Input: part model. Units: mm. Frame: model coordinates. A direction names the side the tool comes from. Coordinates: 2 decimals unless noted, no trailing zeros. Loops run counter-clockwise (first coordinate to the right, second up) from the corner with the lowest first, then second, coordinate; pieces in that order, holes last.
```python
from build123d import *
from build123d.topology import SkipClean

# Parameters (mm, degrees)
SKETCH1_R               = 31
SKETCH1_R_2             = 27.5
BOSS_EXTRUDE1_DEPTH     = 62
BOSS_EXTRUDE3_START     = 5
BOSS_EXTRUDE3_DEPTH     = 5
CUT_EXTRUDE1_DEPTH      = 76.934182026
CUT_EXTRUDE1_DEPTH_BACK = 76.934182026
SKETCH8_W               = 15
SKETCH8_H               = 52
SKETCH9_R               = 13.5
SKETCH9_R_2             = 11
BOSS_EXTRUDE4_DEPTH     = 26
SKETCH10_R              = 13.5
BOSS_EXTRUDE5_DEPTH     = 3
SKETCH12_R              = 1.5
CUT_EXTRUDE2_DEPTH      = 3


with BuildPart() as part:
    # Sketch1 → Boss-Extrude1 (new body)
    with BuildSketch(Plane(origin=(0, 0, 0), x_dir=(1, 0, 0), z_dir=(0, 1, 0))):
        with Locations(Location((0, 0, 0), (0, 0, 270))):
            Circle(SKETCH1_R)
        with Locations(Location((0, 0, 0), (0, 0, 270))):
            Circle(SKETCH1_R_2, mode=Mode.SUBTRACT)
    extrude(amount=BOSS_EXTRUDE1_DEPTH)

    # Sketch6 → Boss-Extrude3 (add)
    with SkipClean():  # the faces are left unmerged after this step: merging them gives an invalid solid
        with BuildSketch(Plane.XZ.offset(BOSS_EXTRUDE3_START)):
            with BuildLine():
                Line((31, 0), (27.5, 0))
                ThreePointArc((27.5, 0), (27.395354198, -2.396782926), (27.082213208, -4.775324886))
                Line((27.082213208, -4.775324886), (30.529040343, -5.383093508))
                ThreePointArc((30.529040343, -5.383093508), (30.882035641, -2.701828025), (31, 0))
            make_face()
            with BuildLine():
                ThreePointArc((27.082213208, 4.775324886), (27.395354198, 2.396782926), (27.5, 0))
                Line((27.5, 0), (31, 0))
                ThreePointArc((31, 0), (30.882035641, 2.701828025), (30.529040343, 5.383093508))
                Line((30.529040343, 5.383093508), (27.082213208, 4.775324886))
            make_face()
        extrude(amount=-BOSS_EXTRUDE3_DEPTH)

    # Sketch8 → Cut-Extrude1 (cut, two sides: drawn at the far end of the back side and taken through both)
    with BuildSketch(Plane.XY.offset(-CUT_EXTRUDE1_DEPTH_BACK)):
        with Locations((0, 31)):
            Rectangle(SKETCH8_W, SKETCH8_H)
    extrude(amount=CUT_EXTRUDE1_DEPTH + CUT_EXTRUDE1_DEPTH_BACK, mode=Mode.SUBTRACT)

    # Sketch9 → Boss-Extrude4 (add)
    with BuildSketch(Plane(origin=(-7.5, 0, 0), x_dir=(0, 0, -1), z_dir=(1, 0, 0))):
        with Locations(Location((41.079062485, 29.5, 0), (0, 0, 270))):
            Circle(SKETCH9_R)
        with Locations((41.079062485, 29.5)):
            Circle(SKETCH9_R_2, mode=Mode.SUBTRACT)
    boss_extrude4 = extrude(amount=-BOSS_EXTRUDE4_DEPTH)

    # Sketch10 → Boss-Extrude5 (add)
    with BuildSketch(Plane.ZY.offset(33.5)):
        with Locations(Location((-41.079062485, 29.5, 0), (0, 0, 270))):
            Circle(SKETCH10_R)
    boss_extrude5 = extrude(amount=BOSS_EXTRUDE5_DEPTH)

    # Sketch12 → Cut-Extrude2 (cut)
    with BuildSketch(Plane(origin=(-17.285590039, -28.448353543, -28.838033475), x_dir=(1, 0, 0), z_dir=(0, 0, 1))):
        with Locations((-14.214409961, 57.948353543)):
            Circle(SKETCH12_R)
    cut_extrude2 = extrude(amount=-CUT_EXTRUDE2_DEPTH, mode=Mode.SUBTRACT)

    # Mirror1: Boss-Extrude4, Boss-Extrude5, Cut-Extrude2 across plane
    add(boss_extrude4.mirror(Plane.XY))
    add(boss_extrude5.mirror(Plane.XY))
    add(cut_extrude2.mirror(Plane.XY), mode=Mode.SUBTRACT)


solid = part.part
```
Item 1: Mould query, pull axis X, two halves, no side actions, for faces 1 (the face through (-20.32, 25.29, 51.24)), 2 (the face through (7.5, 31, 28)), 3 (the face through (-36.5, 30, -41)), 4 (the face through (0, 57, 29)). Classes: +X half, -X half, draft (parallel to the pull), parting line (faces both ways), or undercut.
Result:
face 1: draft
face 2: undercut
face 3: -X half
face 4: undercut
Item 2: Contact query for flat-ended pins moving along their axis: P1, Ø11, axis at y = 34, z = -39, coming from the +X side; P2, Ø3, axis at y = 19, z = -29, coming from the -X side; P3, Ø8, axis at x = 13, y = 54, coming from the +Z side; P4, Ø18.5, axis at x = 0.5, z = 9.5, coming from the -Y side. Output: stop coordinate, or through.
Result:
P1: stops at x = -33.5
P2: stops at x = -14.31
P3: stops at z = 29.66
P4: passes through
Item 3: Reachability of faces 5 (the face through (0, 57, -29)), 6 (the face through (-20.32, 25.29, -51.24)), 7 (the face through (-33, 29.57, 29.5)) from +Z, -Z, +X, -X, +Y, -Y: full face, straight path, thin tool, end or side. Return the list, or none.
Result:
face 5: +Z, -Z
face 6: +X
face 7: none
Item 4: Line query: L1, parallel to Z at x = -9, y = 25.5; L2, parallel to Z at x = -33, y = 25.5; L3, parallel to X at y = 18, z = 0. Output: solid intervals per line, ascending.
Result:
L1: z = -53.97 to -51.33, -30.83 to -25.99, 25.99 to 30.83, 51.33 to 53.97
L2: z = -53.97 to -51.33, -30.83 to -28.19, 28.19 to 30.83, 51.33 to 53.97
L3: x = -31 to -27.5, 27.5 to 31
Item 5: Section query A-A (y = 13). Output: boundary loops of the cut face in (x, z), then the cut area to 3 significant figures.
Result:
outline: (-7.5, -30.08) - (-7.5, -26.46) arc R27.5 cw to (-7.5, 26.46) - (-7.5, 30.08) arc R31 ccw to start; (7.5, -30.08) arc R31 ccw to (7.5, 30.08) - (7.5, 26.46) arc R27.5 cw to (7.5, -26.46) - close
area: 537 mm2
Item 6: Section query D-D (z = 37.5). Output: boundary loops of the cut face in (x, y), then the cut area to 3 significant figures.
Result:
outline: (-36.5, 16.48) - (-7.5, 16.48) - (-7.5, 19.1) - (-33.5, 19.1) - (-33.5, 39.9) - (-7.5, 39.9) - (-7.5, 42.52) - (-36.5, 42.52) - close
area: 214 mm2
Item 7: Section query C-C (y = 3). Output: boundary loops of the cut face in (x, z), then the cut area to 3 significant figures.
Result:
outline: circle Ø62 at (0, 0); hole circle Ø55 at (0, 0)
area: 643 mm2
Item 8: Section query B-B (z = -20.5). Output: boundary loops of the cut face in (x, y).
Result:
outline: (-23.25, 0) - (-18.33, 0) - (-18.33, 62) - (-23.25, 62) - close; (18.33, 0) - (23.25, 0) - (23.25, 62) - (18.33, 62) - close
